Here's the drawing with two shaded views (mm, measured from the low corner). I have some questions. A direction names the side the tool comes from. Coordinates: 2 decimals unless noted, no trailing zeros. Order: outer loops, then holes, each group sorted by start corner. A loop starts at its lowest first (then second) coordinate and runs counter-clockwise, first axis right, second up. Notation, with made-up numbers: (39, 88) -> (83, 88) arc R34 cw to (83, 126) -> close; hole circle Ø3 at (6.5, 59.5). An arc over 180 degrees is marked (long way). One line per item, written item: value. Start each with the question number.
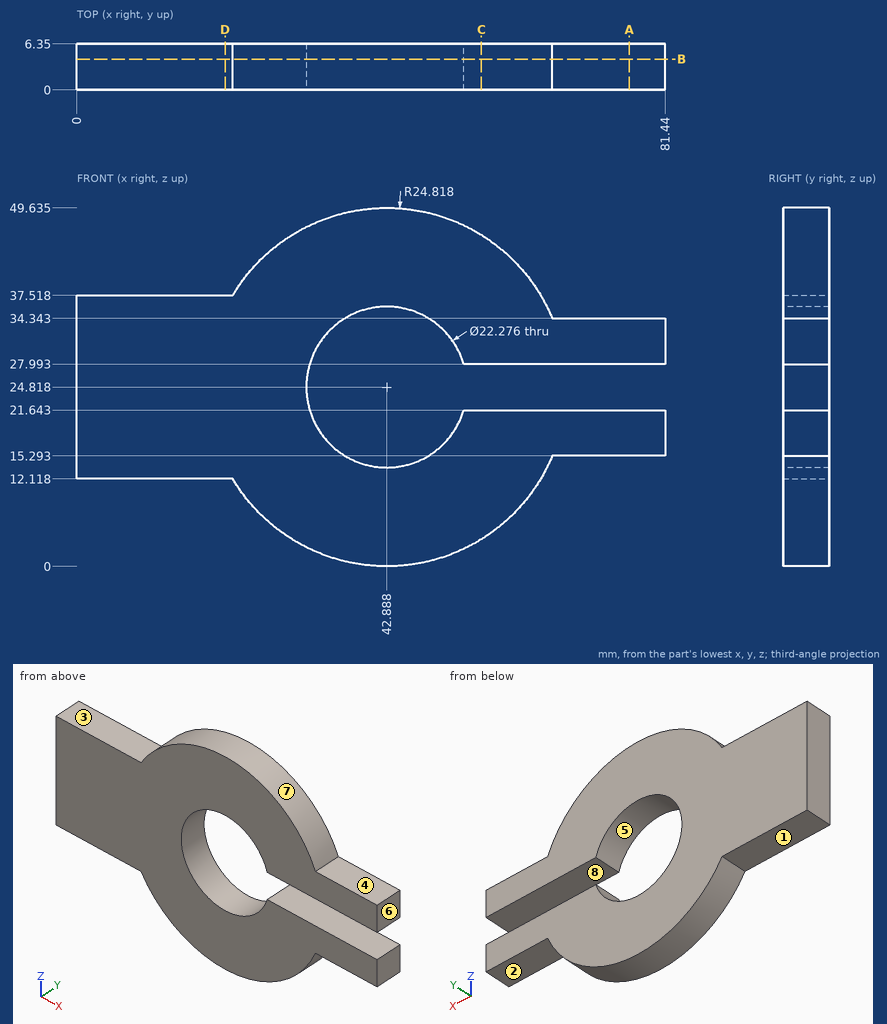
Q1. If we mould it in two halves opening along Z, with no side actions, what happens to the marked faces 5, 6, 7 and 8? For each: +Z half, -Z half, draft (parallel to the pull), parting line (faces both ways), or undercut.
Q2. For P1, Ø1.5, axis at x = 68.5, z = 19, coming from the -Y side; P2, Ø1.5, axis at x = 10.5, z = 38.5, coming from the -Y side; P3, Ø3, axis at x = 10.5, y = 3, coming from the +Z side; P4, Ø1.5, axis at y = 4, z = 38, coming from the +X side, each with a flat end and sliding along its axis, tell me the tip position at first contact or that it passes through.
Q3. Imagine slicing it at C-C (x = 56). Write out the boundary of the cut face in (y, z).
Q4. Imagine slicing it at A-A (x = 76.5). Write out the boundary of the cut face in (y, z).
Q5. Imagine slicing it at B-B (y = 4.25). Write out the boundary of the cut face in (x, z) (1 decimal).
Q6. Imagine slicing it at D-D (x = 20.5). Write out the boundary of the cut face in (y, z), plus the area to 3 significant figures.
Q7. I need wall thicknesses on line 1 (Z direction, x = 70, y = 2.25); line 2 (Z direction, x = 20, y = 3); line 3 (X direction, y = 5, z = 31) (1 decimal). Which ranges of each line are inside material? Lowest first, please.
Q8. For the marked faces 1, 2, 3 and 4, which set-ups out of +Z, -Z, +X, -X, +Y, -Y let a thin tool reach every point of the face, with its end or its side?
Completed:
1. face 5: undercut
1. face 6: draft
1. face 7: +Z half
1. face 8: undercut
2. P1: stops at y = 0
2. P2: passes through
2. P3: stops at z = 37.52
2. P4: stops at x = 64.37
3. outline: (0, 3.75) -> (6.35, 3.75) -> (6.35, 21.64) -> (0, 21.64) -> close; (0, 27.99) -> (6.35, 27.99) -> (6.35, 45.89) -> (0, 45.89) -> close
4. outline: (0, 15.29) -> (6.35, 15.29) -> (6.35, 21.64) -> (0, 21.64) -> close; (0, 27.99) -> (6.35, 27.99) -> (6.35, 34.34) -> (0, 34.34) -> close
5. outline: (0, 12.1) -> (21.6, 12.1) arc R24.8 ccw to (65.8, 15.3) -> (81.4, 15.3) -> (81.4, 21.6) -> (53.6, 21.6) arc R11.1 cw (long way) to (53.6, 28) -> (81.4, 28) -> (81.4, 34.3) -> (65.8, 34.3) arc R24.8 ccw to (21.6, 37.5) -> (0, 37.5) -> close
6. outline: (0, 12.12) -> (6.35, 12.12) -> (6.35, 37.52) -> (0, 37.52) -> close
6. area: 161 mm2
7. line 1: z = 15.29 to 21.64, 27.99 to 34.34
7. line 2: z = 12.12 to 37.52
7. line 3: x = 0 to 33.6, 52.2 to 81.4
8. face 1: -Z, -X, +Y, -Y
8. face 2: -Z, +X, +Y, -Y
8. face 3: +Z, -X, +Y, -Y
8. face 4: +Z, +X, +Y, -Y
